from build123d import *

# Parameters (mm, degrees)
SKETCH2_R           = 45
SKETCH2_R_2         = 18.375
BOSS_EXTRUDE1_DEPTH = 6
SKETCH2_3_R         = 2.575
CUT_EXTRUDE1_DEPTH  = 7
CUT_EXTRUDE3_START  = 6
CUT_EXTRUDE3_DEPTH  = 3.5


with BuildPart() as part:
    # Sketch2 → Boss-Extrude1 (new body)
    with BuildSketch(Plane(origin=(0, 0, 0), x_dir=(1, 0, 0), z_dir=(0, 1, 0))):
        with Locations((0.5741705, -1.235944224)):
            Circle(SKETCH2_R)
        with Locations((0.5741705, -1.235944224)):
            Circle(SKETCH2_R_2, mode=Mode.SUBTRACT)
    extrude(amount=BOSS_EXTRUDE1_DEPTH)

    # Sketch2<3> → Cut-Extrude1 (cut, through all)
    with BuildSketch(Plane(origin=(0, 0, 0), x_dir=(1, 0, 0), z_dir=(0, 1, 0))):
        with Locations((-18.1758295, 31.240008418)):
            Circle(SKETCH2_3_R)
        with Locations((19.3241705, 31.240008418)):
            Circle(SKETCH2_3_R)
        with Locations((38.0741705, -1.235944224)):
            Circle(SKETCH2_3_R)
        with Locations((19.3241705, -33.711896866)):
            Circle(SKETCH2_3_R)
        with Locations((-18.1758295, -33.711896866)):
            Circle(SKETCH2_3_R)
        with Locations((-36.9258295, -1.235944224)):
            Circle(SKETCH2_3_R)
    extrude(amount=CUT_EXTRUDE1_DEPTH, mode=Mode.SUBTRACT)

    # Sketch2<5> → Cut-Extrude3 (cut)
    with BuildSketch(Plane(origin=(0, 0, 0), x_dir=(1, 0, 0), z_dir=(0, 1, 0)).offset(CUT_EXTRUDE3_START)):
        Polygon((22.138316387, 27.577507051), (23.903062668, 31.845879563), (21.088916781, 35.508380929), (16.510024613, 34.902509784), (14.745278332, 30.634137273), (17.559424219, 26.971635906), align=None)
        Polygon((-15.361683613, 27.577507051), (-13.596937332, 31.845879563), (-16.411083219, 35.508380929), (-20.989975387, 34.902509784), (-22.754721668, 30.634137273), (-19.940575781, 26.971635906), align=None)
        Polygon((36.309424219, -5.504316736), (40.888316387, -4.898445591), (42.653062668, -0.630073079), (39.838916781, 3.032428287), (35.260024613, 2.426557142), (33.495278332, -1.841815369), align=None)
        Polygon((14.745278332, -34.317768011), (17.559424219, -37.980269378), (22.138316387, -37.374398233), (23.903062668, -33.106025721), (21.088916781, -29.443524355), (16.510024613, -30.0493955), align=None)
        Polygon((-20.989975387, -30.0493955), (-22.754721668, -34.317768011), (-19.940575781, -37.980269378), (-15.361683613, -37.374398233), (-13.596937332, -33.106025721), (-16.411083219, -29.443524355), align=None)
        Polygon((-35.161083219, 3.032428287), (-39.739975387, 2.426557142), (-41.504721668, -1.841815369), (-38.690575781, -5.504316736), (-34.111683613, -4.898445591), (-32.346937332, -0.630073079), align=None)
    extrude(amount=-CUT_EXTRUDE3_DEPTH, mode=Mode.SUBTRACT)


solid = part.part
Design review of the part built by this model. Coordinates are the model's own, in mm. A direction names the side the tool comes from. Give positions to 0.01 mm unless a question says otherwise; leave off trailing zeros. Write each loop counter-clockwise with the first axis right and the second up, starting at its lowest first coordinate (ties: lowest second). Pieces come first, ordered by that corner, then holes. Notation, with made-up numbers: M -27,0.5 L 30,0.5 A10 cw 30,9.5 Z; hole C -31.75,31 d8. An arc over 180 degrees is marked long. Answer as a JSON object with one key per item and string values. Group by question number.
1) We need section D-D (y = 3.7). Count the separate pieces of the cut face and the enclosed holes in it, and give its area (3 significant figures).
2) For line 1 along X through (y, z) = (5.1, -34.5); line 2 along Z through (x, y) = (19.5, 4.6); line 3 along X through (y, z) = (4.6, -30), list the stretches that pass through material, from the lowest coordinate up.
3) Clearance check with flat-ended pins moving along their axes: pin 1 Ø9.5 at (x, z) = (-38, 1.5) entering from +Y; pin 2 Ø1 at (y, z) = (3.5, -2) entering from -X; pin 3 Ø2.5 at (x, z) = (39.5, 2) entering from +Y; pin 4 Ø1 at (y, z) = (2, 12) entering from +X. State where each tip first meets the part, or that it passes through.
4) Tool access review of faces 1 (the face through (-1.818, 2.958, -16.983)), 2 (the face through (38, 2.5, 4)): name each direction out of +Z, -Z, +X, -X, +Y, -Y from which nothing blocks a thin tool from reaching the whole face with its end or side.
5) We need section B-B (x = 10). Give the boundary of the cut face in (y, z), and give its area (3 significant figures).
6) We need section C-C (z = -24.5). Give the boundary of the cut face in (x, y), and give its area (3 significant figures).
7) We need section A-A (z = 16). Give the boundary of the cut face in (x, y).
Answer key:
{
 "1": {"separate pieces": "1", "enclosed holes": "7", "area": "4,970 mm²"},
 "2": {"line 1": "x = -26.77 to -21.16, -15.64 to 16.34, 21.86 to 27.92", "line 2": "z = -39.59 to -35.3, -27.23 to 29.65, 37.72 to 42.06", "line 3": "x = -31.82 to -22.27, -14.36 to 15.23, 23.14 to 32.97"},
 "3": {"pin 1": "stops at y = 6", "pin 2": "stops at x = -44.34", "pin 3": "stops at y = 2.5", "pin 4": "stops at x = 44.39"},
 "4": {"face 1": "+Y, -Y", "face 2": "+Y"},
 "5": {"outline": "M 0,-42.77 L 6,-42.77 L 6,-14.54 L 0,-14.54 Z; M 0,17.01 L 6,17.01 L 6,45.24 L 0,45.24 Z", "area": "339 mm²"},
 "6": {"outline": "M -36.34,0 L 37.49,0 L 37.49,6 L -36.34,6 Z", "area": "443 mm²"},
 "7": {"outline": "M -41.93,0 L -10.36,0 L -10.36,6 L -41.93,6 Z; M 11.51,0 L 43.08,0 L 43.08,6 L 11.51,6 Z"}
}
